Autodesk Inventor part; units mm, degrees
ref_plane "YZ Plane" through (0, 0, 0) normal (1, 0, 0) x (0, 1, 0)
ref_plane "XZ Plane" through (0, 0, 0) normal (0, 1, 0) x (-1, 0, 0)
ref_plane "XY Plane" through (0, 0, 0) normal (0, 0, 1) x (1, 0, 0)
sketch "Sketch1" plane through (0, 0, 0) normal (0, 0, 1) x (1, 0, 0)
  line L0 (0, 0) -> (33.49, 0)
  line L1 (33.49, 0) -> (33.49, 58.49)
  line L2 (33.49, 58.49) -> (0, 58.49)
  line L3 (0, 58.49) -> (0, 0)
  line L4 (-2, 60.49) -> (35.49, 60.49)
  line L5 (35.49, 60.49) -> (35.49, -2)
  line L6 (35.49, -2) -> (-2, -2)
  line L7 (-2, -2) -> (-2, 60.49)
  dimension "d0" = 33.49
  dimension "d1" = 58.49
  dimension "d2" = 2
extrude "Extrusion1" add sketch "Sketch1" along normal blind 46
sketch "Sketch2" plane through (0, 0, 46) normal (0, 0, 1) x (1, 0, 0)
  line L0 (-2, 60.49) -> (-2, -2)
  line L1 (-2, 0) -> (35.49, 0)
  line L2 (35.49, -2) -> (35.49, 60.49)
  line L3 (-2, -2) -> (35.49, -2)
  line L4 (35.49, -2) -> (-2, -2)
  line L5 (-2, -2) -> (-2, 0)
  point P0 (0, 0)
extrude "Extrusion2" cut sketch "Sketch2" against normal blind 32
sketch "Sketch3" plane through (0, 0, 0) normal (0, 0, -1) x (-1, 0, 0)
  line L0 (-35.49, 60.49) -> (2, 60.49)
  line L1 (2, -2) -> (-35.49, -2)
  line L2 (-35.49, 60.49) -> (2, 60.49)
  line L3 (2, 60.49) -> (2, -2)
  line L4 (2, -2) -> (-35.49, -2)
  line L5 (-35.49, -2) -> (-35.49, 60.49)
  point P0 (0, 0)
extrude "Extrusion3" add sketch "Sketch3" along normal blind 2
sketch "Sketch4" plane through (-2, 0, 46) normal (-1, 0, 0) x (0, 0, 1)
  line L0 (-48, -2) -> (-48, 60.49)
  line L1 (-48, 35.745) -> (-42, 35.745)
  line L2 (-42, 35.745) -> (-42, 22.745)
  line L3 (-42, 22.745) -> (-48, 22.745)
  line L4 (-48, 60.49) -> (0, 60.49)
  line L5 (-46, 35.745) -> (-46, 22.745)
  point P0 (-46, 0)
  point P1 (-45, 22.745)
  point P2 (-45, 35.745)
  dimension "d10" = 6
  dimension "d11" = 13
  dimension "d12" = 24.745
  dimension "d13" = 2
extrude "Extrusion4" cut sketch "Sketch4" against normal up to surface (37.49 mm away) contours L5 L1 L2 L3
properties part number "Motor_Base_3"
Read the model definition and answer for the solid it produces. Units are mm, in the model's axes. A direction names the side the tool comes from. Give positions to 0.01 mm unless a question says otherwise; leave off trailing zeros. Loops run counter-clockwise (first coordinate to the right, second up) from the corner with the lowest first, then second, coordinate; pieces in that order, holes last.
Item 1: For faces 1 (the flat face through (34, 29, 4)), 2 (the flat face through (16, -2, 6)), 3 (the flat face through (35.49, 29, 22)), 4 (the flat face through (17, 0, 7)), 5 (the flat face through (34, 0, 30)), determine the directions among +Z, -Z, +X, -X, +Y, -Y from which every point of the face is accessible in a straight line to the end or side of a thin tool.
Item 2: The mould has two halves that part along Z. Classify faces 6 (the flat face through (17, 58.49, 23)), 7 (the flat face through (-1, 29, 4)), 8 (the flat face through (-1, 37, 46)): released by +Z, released by -Z, zero draft, split by the parting line, or undercut.
Item 3: Each of these flat-tipped pins is pushed along its axis until it touches: pin 1 Ø1 at (x, y) = (23.5, -0.5) entering from +Z; pin 2 Ø12 at (x, z) = (13.5, 32) entering from -Y; pin 3 Ø0.6 at (x, z) = (-1.5, 27) entering from -Y. Where does it stop, or does it pass through?
Item 4: Find the intervals of material crossed by line 1 along X through (y, z) = (7, 40.5); line 2 along Y through (x, z) = (7, 2); line 3 along Z through (x, y) = (28.5, 13), in increasing order.
Item 5: The part is cut by section A-A (z = 2.5). Write down the section's boundary in (x, y) (3 decimals).
Item 6: The part is cut by section D-D (y = 51). Write down the section's boundary in (x, z).
Item 7: The part is cut by section B-B (y = 33). Write down the section's boundary in (x, z), and give its area (3 significant figures).
Item 8: The part is cut by section C-C (z = 11). Write down the section's boundary in (x, y).
Taken from the geometry:
1. face 1: +X, -X
1. face 2: +Z, -Z, +X, -X, -Y
1. face 3: +Z, -Z, +X, +Y, -Y
1. face 4: +Z
1. face 5: +Z, +X, -X, -Y
2. face 6: zero draft
2. face 7: undercut
2. face 8: released by +Z
3. pin 1: stops at z = 14
3. pin 2: stops at y = 58.49
3. pin 3: stops at y = 0
4. line 1: x = -2 to 0, 33.49 to 35.49
4. line 2: y = -2 to 0, 58.49 to 60.49
4. line 3: z = -2 to 0
5. outline: (-2, -2) - (35.49, -2) - (35.49, 22.745) - (33.49, 22.745) - (33.49, 0) - (0, 0) - (0, 22.745) - (-2, 22.745) - close; (-2, 35.745) - (0, 35.745) - (0, 58.49) - (33.49, 58.49) - (33.49, 35.745) - (35.49, 35.745) - (35.49, 60.49) - (-2, 60.49) - close
6. outline: (-2, -2) - (35.49, -2) - (35.49, 46) - (33.49, 46) - (33.49, 0) - (0, 0) - (0, 46) - (-2, 46) - close
7. outline: (-2, -2) - (35.49, -2) - (35.49, 0) - (-2, 0) - close; (-2, 4) - (0, 4) - (0, 46) - (-2, 46) - close; (33.49, 4) - (35.49, 4) - (35.49, 46) - (33.49, 46) - close
7. area: 243 mm2
8. outline: (-2, -2) - (35.49, -2) - (35.49, 60.49) - (-2, 60.49) - close; hole (0, 0) - (33.49, 0) - (33.49, 58.49) - (0, 58.49) - close
